Geometry check sheet. Reference: the model listing, model coordinates, mm. A direction names the side the tool comes from. Round coordinates to 2 decimals unless told otherwise and drop trailing zeros. Order: outer loops, then holes, each group sorted by start corner. A loop starts at its lowest first (then second) coordinate and runs counter-clockwise, first axis right, second up. Notation, with made-up numbers: (27.5, -38.75) - (83.5, -38.75) arc R29 ccw to (83.5, -17.75) - close; hole circle Ø3 at (61.5, -32). An arc over 180 degrees is marked (long way). Use a Markdown table: item, result. Add a question column.
(1) Mould release check, pull along Z, two halves, no side actions. Record for faces 1 (the face through (2.75, 1.52, 3.08)), 2 (the face through (-10, 2, 16)), 3 (the face through (-15, 1, -19)): released by +Z, released by -Z, zero draft, split by the parting line, or undercut.
(2) Section check C-C on z = 1.5. Record the boundary of the cut face in (x, y).
(3) Access from +Z, -Z, +X, -X, +Y, -Y to the whole of each face (thin tool, end or side, straight path). Record for faces 4 (the face through (-5, 1, -19)), 5 (the face through (-3, 2, -1.788)), 6 (the face through (13, 2, 18)), 7 (the face through (0, 2, -16)).
(4) Section check A-A on x = -4.5. Record the boundary of the cut face in (y, z), then the cut area to 3 significant figures.
(5) Gauge pin test, flat ends, axial feed: P1, Ø5, axis at x = -11.5, z = -13, coming from the -Y side; P2, Ø1, axis at x = -8, y = 1, coming from the -Z side. Record the tip position at first contact, or that the pin passes through.
(6) Thickness scan on line 1 along X through (y, z) = (0.7, -16.5); line 2 along Z through (x, y) = (-5.5, 1.1); line 3 along Z through (x, y) = (-10.5, 0.8). Record the ranges inside material, lowest first. Write a range as [from, to].
```python
from build123d import *

# Parameters (mm, degrees)
SKETCH1_W            = 34
SKETCH1_H            = 38
BOSS_EXTRUDE1_DEPTH  = 3
SKETCH3_W            = 6
SKETCH3_H            = 3
CUT_EXTRUDE2_DEPTH   = 3
LPATTERN2_COUNT      = 3
LPATTERN2_PITCH      = 10
LPATTERN2_COUNT_DIR2 = 2
LPATTERN2_PITCH_DIR2 = 35
CUT_EXTRUDE4_DEPTH   = 3


with BuildPart() as part:
    # Sketch1 → Boss-Extrude1 (new body)
    with BuildSketch(Plane(origin=(0, 0, 0), x_dir=(1, 0, 0), z_dir=(0, 1, 0))):
        Rectangle(SKETCH1_W, SKETCH1_H)
    extrude(amount=BOSS_EXTRUDE1_DEPTH)

    # Sketch3 → Cut-Extrude2 (cut)
    with BuildSketch(Plane(origin=(0, 3, 0), x_dir=(1, 0, 0), z_dir=(0, 1, 0))):
        with Locations((-10, 17.5)):
            Rectangle(SKETCH3_W, SKETCH3_H)
    cut_extrude2 = extrude(amount=-CUT_EXTRUDE2_DEPTH, mode=Mode.SUBTRACT)

    # LPattern2: Cut-Extrude2 3 × 2
    with Locations(*[(i * LPATTERN2_PITCH, 0, j * LPATTERN2_PITCH_DIR2) for i in range(LPATTERN2_COUNT) for j in range(LPATTERN2_COUNT_DIR2) if (i, j) != (0, 0)]):
        add(cut_extrude2, mode=Mode.SUBTRACT)

    # Sketch4 → Cut-Extrude4 (cut)
    with BuildSketch(Plane(origin=(0, 3, 0), x_dir=(1, 0, 0), z_dir=(0, 1, 0))):
        with BuildLine():
            Line((-6.178432091, -7.791666667), (0.178432091, -7.791666667))
            ThreePointArc((0.178432091, -7.791666667), (2.74999925, -3.002936198), (0.183324096, 1.788418079))
            Line((0.183324096, 1.788418079), (-6.183324096, 1.788418079))
            ThreePointArc((-6.183324096, 1.788418079), (-8.74999925, -3.002936198), (-6.178432091, -7.791666667))
        make_face()
    extrude(amount=-CUT_EXTRUDE4_DEPTH, mode=Mode.SUBTRACT)


solid = part.part
```
Check sheet entries:
| question | item | result |
|---|---|---|
| 1 | face 1 | undercut |
| 1 | face 2 | released by +Z |
| 1 | face 3 | released by -Z |
| 2 | outline | (-17, 0) - (-8.55, 0) - (-8.55, 3) - (-17, 3) - close; (2.55, 0) - (17, 0) - (17, 3) - (2.55, 3) - close |
| 3 | face 4 | -Z, +X, -X, +Y, -Y |
| 3 | face 5 | +Y, -Y |
| 3 | face 6 | +Z, +Y, -Y |
| 3 | face 7 | -Z, +Y, -Y |
| 4 | outline | (0, -19) - (3, -19) - (3, -1.79) - (0, -1.79) - close; (0, 7.79) - (3, 7.79) - (3, 19) - (0, 19) - close |
| 4 | area | 85.3 mm2 |
| 5 | P1 | stops at y = 0 |
| 5 | P2 | stops at z = -16 |
| 6 | line 1 | x = [-17, -13], [-7, -3], [3, 7], [13, 17] |
| 6 | line 2 | z = [-19, -1.79], [7.79, 19] |
| 6 | line 3 | z = [-16, 16] |
